from build123d import *

# Parameters (mm, degrees)
F0_R     = 38.1
F0_R_2   = 6.35
F1_DEPTH = 12.7
F2_R     = 6.35
F2_R_2   = 3.810001
F2_R_3   = 3.81
F3_DEPTH = 12.7
F4_R     = 2.54
F5_SIZE  = 2.54


with BuildPart() as f1:
    # F0 (on Top) → F1 (new body)
    with BuildSketch(Plane.XY):
        Circle(F0_R)
        with Locations((-16.948049, -23.936937)):
            Circle(F0_R_2, mode=Mode.SUBTRACT)
        with Locations((29.20402, -2.708972)):
            Circle(F0_R_2, mode=Mode.SUBTRACT)
        with Locations((-12.255971, 26.64591)):
            Circle(F0_R_2, mode=Mode.SUBTRACT)
    extrude(amount=F1_DEPTH)

    # F2 (on face) → F3 (join)
    with BuildSketch(Plane.XY.offset(12.7)):
        with Locations((-16.948049, -23.936937)):
            Circle(F2_R)
        with Locations((-16.948049, -23.936937)):
            Circle(F2_R_2, mode=Mode.SUBTRACT)
        with Locations((-12.255971, 26.64591)):
            Circle(F2_R)
        with Locations((-12.255971, 26.64591)):
            Circle(F2_R_3, mode=Mode.SUBTRACT)
        with Locations((29.20402, -2.708972)):
            Circle(F2_R)
        with Locations((29.20402, -2.708972)):
            Circle(F2_R_3, mode=Mode.SUBTRACT)
    extrude(amount=-F3_DEPTH)

    # F4
    f4_edges = [f1.edges().sort_by_distance(p)[0] for p in [
        (25.39402, -2.708972, 0),
        (-16.065971, 26.64591, 0),
        (-20.75805, -23.936937, 0),
    ]]
    fillet(f4_edges, radius=F4_R)

    # F5
    f5_edges = [f1.edges().sort_by_distance(p)[0] for p in [
        (-16.065971, 26.64591, 12.7),
        (25.39402, -2.708972, 12.7),
        (-20.75805, -23.936937, 12.7),
    ]]
    chamfer(f5_edges, length=F5_SIZE)


solid = f1.part
Design review of the part built by this model. Coordinates are the model's own, in mm. Coordinates: 2 decimals unless noted, no trailing zeros. Loops run counter-clockwise (first coordinate to the right, second up) from the corner with the lowest first, then second, coordinate; pieces in that order, holes last.
Item 1: Wall thickness on L1, parallel to Y at x = -15.5, z = 6.75; L2, parallel to X at y = -25.5, z = 6.75; L3, parallel to Y at x = -18, z = 5: over which ranges is each line inside the solid? List them lowest first.
Completed:
L1: y = -34.8 to -27.46, -20.41 to 24.65, 28.64 to 34.8
L2: x = -28.31 to -20.42, -13.47 to 28.31
L3: y = -33.58 to -27.6, -20.28 to 33.58
Item 2: Add section A-A (z = 4.5). Write out the cut boundary in (x, y), and give its area (3 significant figures).
Completed:
outline: circle Ø76.2 at (0, 0); hole circle Ø7.62 at (-16.95, -23.94); hole circle Ø7.62 at (-12.26, 26.65); hole circle Ø7.62 at (29.2, -2.71)
area: 4,420 mm2
Item 3: Add section C-C (y = -13). Write out the cut boundary in (x, z).
Completed:
outline: (-35.81, 0) - (35.81, 0) - (35.81, 12.7) - (-35.81, 12.7) - close
Item 4: Clearance check with flat-ended pins moving along their axes: pin 1 (6 mm diameter, centred on x = -13, z = 6.5, fed in from -Y); pin 2 (2 mm diameter, centred on x = -6, z = 7, fed in from -Y); pin 3 (5 mm diameter, centred on x = 25, z = 5, fed in from -Y). State where each tip first meets the part, or that it passes through.
Completed:
pin 1: stops at y = -36.76
pin 2: stops at y = -37.77
pin 3: stops at y = -30.75
Item 5: Add section B-B (y = 19). Write out the cut boundary in (x, z), and give its area (3 significant figures).
Completed:
outline: (-33.02, 0) - (33.02, 0) - (33.02, 12.7) - (-33.02, 12.7) - close
area: 839 mm2
Item 6: Draft analysis for pull direction Y (two halves, no side actions). For faces 1 (the cylindrical face through (-15.064, 29.221, 6.403)), 2 (the conical face through (32.837, -4.215, 10.283)), 3 (the flat face through (-1, 1, 0)), 4 (the cylindrical face through (-30.235, -23.183, 6.261)), state which applies: pulls with the +Y half, pulls with the -Y half, needs draft (parallel to the pull), parting line crosses it, or undercut.
Completed:
face 1: undercut
face 2: undercut
face 3: needs draft
face 4: parting line crosses it
